Can you work these out from the model? Positions are in its coordinate system, mm. A direction names the side the tool comes from. Round coordinates to 2 decimals unless told otherwise and drop trailing zeros. Order: outer loops, then holes, each group sorted by start corner. A loop starts at its lowest first (then second) coordinate and runs counter-clockwise, first axis right, second up.
from build123d import *

# Parameters (mm, degrees)
F0_R     = 20
F1_DEPTH = 10
F3_DEPTH = 2
F4_COUNT = 7


with BuildPart() as f1:
    # F0 (on Top) → F1 (new body)
    with BuildSketch(Plane.XY):
        Circle(F0_R)
    extrude(amount=F1_DEPTH)

    # F2 (on face) → F3 (join)
    with BuildSketch(Plane.XY.offset(10)):
        with BuildLine():
            Line((1.5, 15.929532), (1.5, 19.943671))
            ThreePointArc((1.5, 19.943671), (0, 20), (-1.5, 19.943671))
            Line((-1.5, 19.943671), (-1.5, 15.929532))
            ThreePointArc((-1.5, 15.929532), (0, 16), (1.5, 15.929532))
        make_face()
    extrude(amount=F3_DEPTH)

    # F4: F1 ×7 about axis
    f4_axis = Axis((0, 0, 0), (0, 0, -1))


with BuildPart() as f1_1:
    add(f1.part)
    for i in range(1, F4_COUNT):
        add(f1.part.rotate(f4_axis, i * 360 / F4_COUNT))


solid = f1_1.part
(1) Please list where these lines run through material, in increasing order: probe 1 along X at (y, z) = (-13, 3.25); probe 2 along Y at (x, z) = (-16, 10.5); probe 3 along Y at (x, z) = (0, 2.25).
(2) On a 3-axis mill with a long thin cutter (end or side, diameter ignored), from which of +Z, -Z, +X, -X, +Y, -Y can I reach the whole of each face in a straight line? I mean faces 1 (the face through (9.146, -15.535, 10.986)), 2 (the face through (6.42, -16.79, 10.99)), 3 (the face through (15.604, -3.54, 10.986)). Say none if no direction works.
(3) I want a section at A-A, the plane x = 0. List the corners of the cut face in (y, z) for me, plus the area to 3 significant figures.
(4) If we mould it in two halves opening along X, with no side actions, what happens to faces 4 (the face through (6.961, -14.406, 10.986)), 5 (the face through (-14, 11, 12)), 6 (the face through (19.494, -4.471, 10.986))? For each: pulls with the +X half, pulls with the -X half, needs draft (parallel to the pull), parting line crosses it, or undercut.
(5) I want a section at B-B, the plane z = 6.5. List the corners of the cut face in (x, y) for me.
(6) I want a section at C-C, the plane y = 10.5. List the corners of the cut face in (x, z) for me, plus the area to 3 significant figures.
(7) I'm going to push flat-ended pins straight in: pin 1 Ø4 at (y, z) = (5.5, 7.5) entering from +X; pin 2 Ø12 at (x, y) = (0.5, -6) entering from +Z; pin 3 Ø10 at (x, y) = (-1.5, 7.5) entering from -Z; pin 4 Ø1.6 at (y, z) = (19, 11) entering from -X. Where does each tip first touch, or does it pass through?
(8) I want a section at D-D, the plane x = -9.5. List the corners of the cut face in (y, z) for me, plus the area to 3 significant figures.
Ans:
1. probe 1: x = -15.2 to 15.2
1. probe 2: y = -5.19 to -2.11, 10.84 to 12
1. probe 3: y = -20 to 20
2. face 1: +Z, +X, +Y
2. face 2: +Z, -Y
2. face 3: +Z
3. outline: (-20, 0) - (20, 0) - (20, 12) - (16, 12) - (16, 10) - (-20, 10) - close
3. area: 408 mm2
4. face 4: undercut
4. face 5: needs draft
4. face 6: pulls with the +X half
5. outline: circle Ø40 at (0, 0)
6. outline: (-17.02, 0) - (17.02, 0) - (17.02, 10) - (15.57, 10) - (15.57, 12) - (12.07, 12) - (12.07, 10) - (-12.07, 10) - (-12.07, 12) - (-15.57, 12) - (-15.57, 10) - (-17.02, 10) - close
6. area: 354 mm2
7. pin 1: stops at x = 19.69
7. pin 2: stops at z = 10
7. pin 3: stops at z = 0
7. pin 4: stops at x = -1.5
8. outline: (-17.6, 0) - (17.6, 0) - (17.6, 10) - (-16.27, 10) - (-16.27, 12) - (-17.6, 12) - close
8. area: 355 mm2
